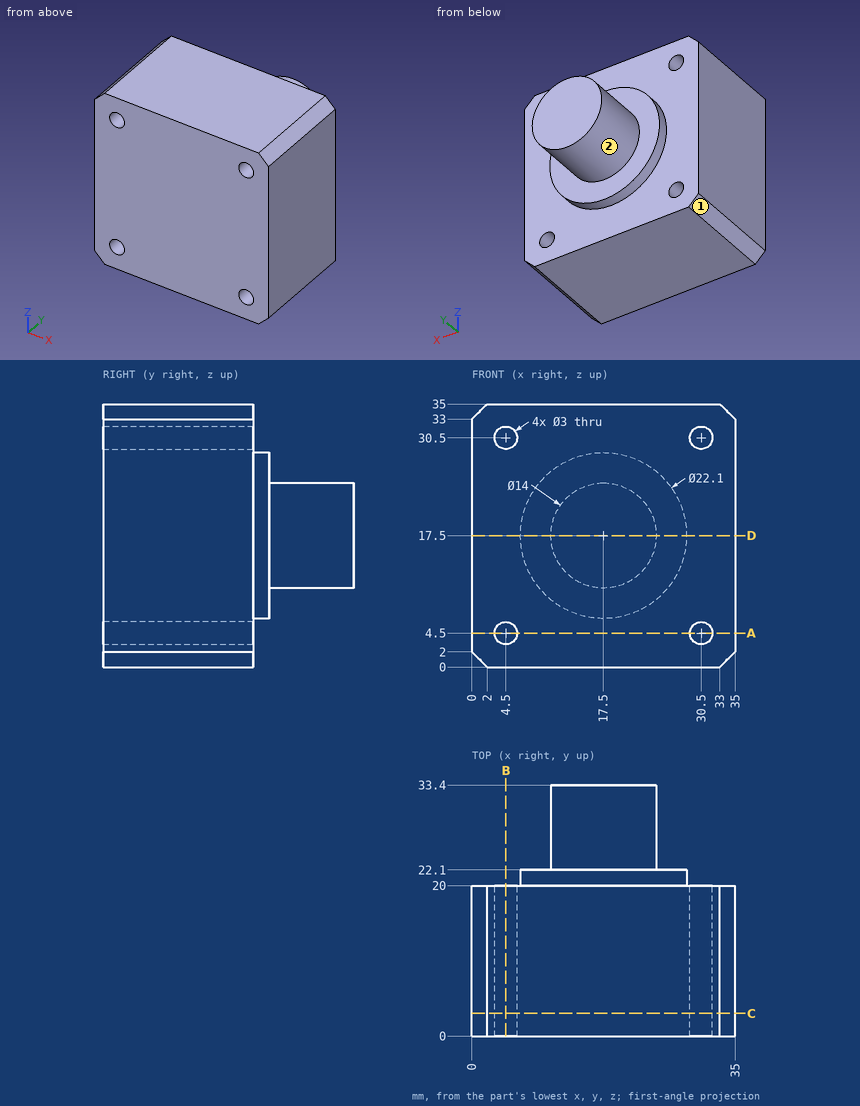
Geometry: see drawing. Coordinates: mm, zero at the bounding-box minimum. A direction names the side the tool comes from. Give positions to 0.01 mm unless a question says otherwise; leave off trailing zeros. Write each loop counter-clockwise with the first axis right and the second up, starting at its lowest first coordinate (ties: lowest second). Pieces come first, ordered by that corner, then holes. Notation, with made-up numbers: M -26.5,73.5 L 1.5,73.5 A13 ccw 1.5,88.5 Z; hole C 66,-20 d3. An arc over 180 degrees is marked long. Answer in a Markdown table with one row per item. Add a question column.
(1) First-contact query: pin 1 (3 mm diameter, centred on x = 21, z = 15.5, fed in from -Y); pin 2 (3.5 mm diameter, centred on x = 4.5, z = 30.5, fed in from +Y). Flat tips, straight axial feed; report the tip coordinate or a pass-through.
(2) Reachability of the marked faces 1 and 2 from +Z, -Z, +X, -X, +Y, -Y: full face, straight path, thin tool, end or side. Return the list, or none.
(3) Ray query, line 1 (X direction, y = 14, z = 4.5); line 2 (X direction, y = 9, z = 30). Return the intervals inside material, ascending.
(4) Section B-B on x = 4.5. Return loops of the section in (y, z), and give its area (3 significant figures).
(5) Section D-D on z = 17.5. Return loops of the section in (x, y).
(6) Section C-C on y = 3. Return loops of the section in (x, z).
(7) Section A-A on z = 4.5. Return loops of the section in (x, y).
Result set:
| question | item | result |
|---|---|---|
| 1 | pin 1 | stops at y = 0 |
| 1 | pin 2 | stops at y = 20 |
| 2 | face 1 | -Z, -X, +Y, -Y |
| 2 | face 2 | +Y |
| 3 | line 1 | x = 0 to 3, 6 to 29, 32 to 35 |
| 3 | line 2 | x = 0 to 3.09, 5.91 to 29.09, 31.91 to 35 |
| 4 | outline | M 0,0 L 20,0 L 20,3 L 0,3 Z; M 0,6 L 20,6 L 20,29 L 0,29 Z; M 0,32 L 20,32 L 20,35 L 0,35 Z |
| 4 | area | 580 mm^2 |
| 5 | outline | M 0,0 L 35,0 L 35,20 L 28.55,20 L 28.55,22.1 L 24.5,22.1 L 24.5,33.4 L 10.5,33.4 L 10.5,22.1 L 6.45,22.1 L 6.45,20 L 0,20 Z |
| 6 | outline | M 0,2 L 2,0 L 33,0 L 35,2 L 35,33 L 33,35 L 2,35 L 0,33 Z; hole C 4.5,4.5 d3; hole C 4.5,30.5 d3; hole C 30.5,4.5 d3; hole C 30.5,30.5 d3 |
| 7 | outline | M 0,0 L 3,0 L 3,20 L 0,20 Z; M 6,0 L 29,0 L 29,20 L 6,20 Z; M 32,0 L 35,0 L 35,20 L 32,20 Z |
